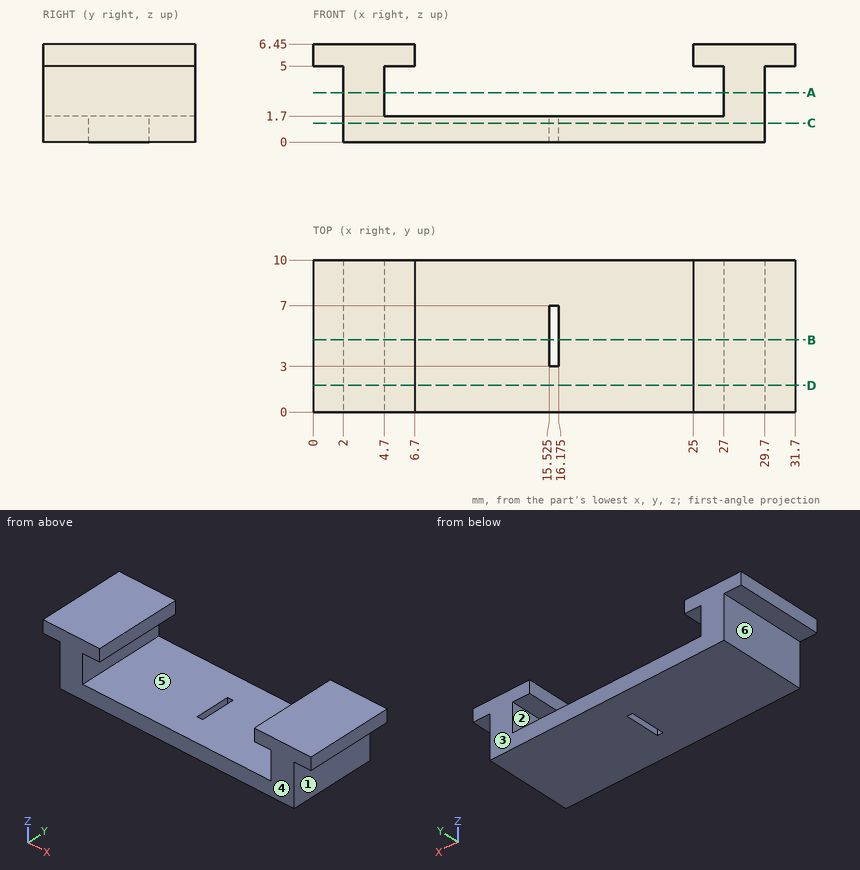
Here's the drawing with two shaded views (mm, measured from the low corner). I have some questions. A direction names the side the tool comes from. Round coordinates to 2 decimals unless told otherwise and drop trailing zeros. Write each loop counter-clockwise with the first axis right and the second up, starting at its lowest first coordinate (ties: lowest second). Pieces come first, ordered by that corner, then holes. Notation, with made-up numbers: M -19,44.25 L -8,44.25 A18 cw -8,70.25 Z; hole C 47.25,61 d5. An arc over 180 degrees is marked long. Answer in a Markdown table with one row per item. Add a question column.
Q1. Imagine slicing it at C-C (z = 1.25). Please give me the cut outline in (x, y) (3 decimals), then the cut area to 3 significant figures.
Q2. Imagine slicing it at A-A (z = 3.25). Please give me the cut outline in (x, y).
Q3. On a 3-axis mill with a long thin cutter (end or side, diameter ignored), from which of +Z, -Z, +X, -X, +Y, -Y can I reach the whole of each face in a straight line? I mean the marked faces 4, 5 and 6. Say none if no direction works.
Q4. If we mould it in two halves opening along X, with no side actions, what happens to the marked faces 1, 2 and 3? For each: +X half, -X half, draft (parallel to the pull), parting line (faces both ways), or undercut.
Q5. Imagine slicing it at D-D (y = 1.75). Please give me the cut outline in (x, z), then the cut area to 3 significant figures.
Q6. Will these pins go through, and if not, where does the flat tip stop? pin 1 Ø1.4 at (y, z) = (4.5, 1) entering from +X; pin 2 Ø0.6 at (x, y) = (31, 3) entering from -Z; pin 3 Ø1.4 at (y, z) = (6, 0.5) entering from -X.
Q7. Imagine slicing it at B-B (y = 4.75). Please give me the cut outline in (x, z) (3 decimals), then the cut area to 3 significant figures.
Q8. If I drill on line 1 (X direction, y = 3.25, z = 3.75); line 2 (X direction, y = 3.25, z = 0.5) (3 decimals); line 3 (Z direction, x = 8.5, y = 5.5), over which ranges is the centre line in solid material (lowest first)? Write a range as from..to.
Values:
| question | item | result |
|---|---|---|
| 1 | outline | M 2,0 L 29.7,0 L 29.7,10 L 2,10 Z; hole M 15.525,3 L 16.175,3 L 16.175,7 L 15.525,7 Z |
| 1 | area | 274 mm^2 |
| 2 | outline | M 2,0 L 4.7,0 L 4.7,10 L 2,10 Z; M 27,0 L 29.7,0 L 29.7,10 L 27,10 Z |
| 3 | face 4 | +Z, -Z, +X, -X, -Y |
| 3 | face 5 | +Y, -Y |
| 3 | face 6 | -Z, -X, +Y, -Y |
| 4 | face 1 | +X half |
| 4 | face 2 | undercut |
| 4 | face 3 | draft |
| 5 | outline | M 0,5 L 2,5 L 2,0 L 29.7,0 L 29.7,5 L 31.7,5 L 31.7,6.45 L 25,6.45 L 25,5 L 27,5 L 27,1.7 L 4.7,1.7 L 4.7,5 L 6.7,5 L 6.7,6.45 L 0,6.45 Z |
| 5 | area | 84.3 mm^2 |
| 6 | pin 1 | x = 29.7 |
| 6 | pin 2 | z = 5 |
| 6 | pin 3 | x = 2 |
| 7 | outline | M 0,5 L 2,5 L 2,0 L 15.525,0 L 15.525,1.7 L 4.7,1.7 L 4.7,5 L 6.7,5 L 6.7,6.45 L 0,6.45 Z; M 16.175,0 L 29.7,0 L 29.7,5 L 31.7,5 L 31.7,6.45 L 25,6.45 L 25,5 L 27,5 L 27,1.7 L 16.175,1.7 Z |
| 7 | area | 83.2 mm^2 |
| 8 | line 1 | 2..4.7, 27..29.7 |
| 8 | line 2 | 2..15.525, 16.175..29.7 |
| 8 | line 3 | 0..1.7 |
